Here's how the part is built. I have some questions about the finished solid (model axes, mm). Face numbers are marked on the shaded views. A direction names the side the tool comes from. Give positions to 0.01 mm unless a question says otherwise; leave off trailing zeros. Loops run counter-clockwise (first coordinate to the right, second up) from the corner with the lowest first, then second, coordinate; pieces in that order, holes last. Notation, with made-up numbers: (43, 35) - (65, 35) arc R14 cw to (65, 45) - close; hole circle Ø2 at (16.25, 76). An arc over 180 degrees is marked (long way). Use one line per item in the form item = value.
from build123d import *

# Parameters (mm, degrees)
SKETCH_2_R          = 23.5
EXTRUDE_1_DEPTH     = 50
FILLET_3_R          = 10
SHELL_2_T           = -2
SKETCH_5_R          = 9.5
EXTRUDE_2_DEPTH     = 48
SKETCH_6_R          = 2.4
CUT_EXTRUDE_1_DEPTH = 61.037488289
EXTRUDE_3_REACH     = 62.037
SKETCH_7_W          = 1.2
SKETCH_7_H          = 13
SKETCH_8_R          = 7.5
CUT_EXTRUDE_2_DEPTH = 39
CHAMFER_1_SIZE      = 3


with BuildPart() as part:
    # Эскиз2 → Бобышка-Вытянуть1 (new body)
    with BuildSketch(Plane.XY):
        Circle(SKETCH_2_R)
    extrude(amount=EXTRUDE_1_DEPTH)

    # Скругление3
    fillet_3_edges = [part.edges().sort_by_distance(p)[0] for p in [
        (-23.5, 0, 50),
    ]]
    fillet(fillet_3_edges, radius=FILLET_3_R)

    # Оболочка2
    shell_2_openings = [part.faces().sort_by_distance(p)[0] for p in [
        (0, 0, 0),
    ]]
    offset(amount=SHELL_2_T, openings=shell_2_openings, kind=Kind.INTERSECTION)

    # Эскиз5 → Бобышка-Вытянуть2 (add)
    with BuildSketch(Plane(origin=(0, 0, 48), x_dir=(-1, 0, 0), z_dir=(0, 0, -1))):
        with Locations(Location((0, 0, 0), (0, 0, 180))):
            Circle(SKETCH_5_R)
    extrude(amount=EXTRUDE_2_DEPTH)

    # Эскиз6 → Вырез-Вытянуть1 (cut, through all)
    with BuildSketch(Plane(origin=(0, 0, 0), x_dir=(-1, 0, 0), z_dir=(0, 0, -1))):
        Circle(SKETCH_6_R)
    extrude(amount=-CUT_EXTRUDE_1_DEPTH, mode=Mode.SUBTRACT)

    # Эскиз7 → Бобышка-Вытянуть3 (add, up to next)
    with BuildSketch(Plane(origin=(0, 0, 0), x_dir=(-1, 0, 0), z_dir=(0, 0, -1)), mode=Mode.PRIVATE) as extrude_3_sk1:
        with Locations((0, 15.437627965)):
            Rectangle(SKETCH_7_W, SKETCH_7_H)
    extrude_3_tool1 = extrude(extrude_3_sk1.sketch, amount=-EXTRUDE_3_REACH, mode=Mode.PRIVATE) - part.part
    # Эскиз7 → Бобышка-Вытянуть3 (add, up to next)
    with BuildSketch(Plane(origin=(0, 0, 0), x_dir=(-1, 0, 0), z_dir=(0, 0, -1)), mode=Mode.PRIVATE) as extrude_3_sk2:
        Polygon((7.440212867, 4.988429225), (18.698543116, 11.488429225), (19.298543116, 10.44919874), (8.040212867, 3.94919874), align=None)
    extrude_3_tool2 = extrude(extrude_3_sk2.sketch, amount=-EXTRUDE_3_REACH, mode=Mode.PRIVATE) - part.part
    # Эскиз7 → Бобышка-Вытянуть3 (add, up to next)
    with BuildSketch(Plane(origin=(0, 0, 0), x_dir=(-1, 0, 0), z_dir=(0, 0, -1)), mode=Mode.PRIVATE) as extrude_3_sk3:
        Polygon((8.040212867, -3.94919874), (19.298543117, -10.44919874), (18.698543117, -11.488429225), (7.440212867, -4.988429225), align=None)
    extrude_3_tool3 = extrude(extrude_3_sk3.sketch, amount=-EXTRUDE_3_REACH, mode=Mode.PRIVATE) - part.part
    # Эскиз7 → Бобышка-Вытянуть3 (add, up to next)
    with BuildSketch(Plane(origin=(0, 0, 0), x_dir=(-1, 0, 0), z_dir=(0, 0, -1)), mode=Mode.PRIVATE) as extrude_3_sk4:
        with Locations((0, -15.437627965)):
            Rectangle(SKETCH_7_W, SKETCH_7_H)
    extrude_3_tool4 = extrude(extrude_3_sk4.sketch, amount=-EXTRUDE_3_REACH, mode=Mode.PRIVATE) - part.part
    # Эскиз7 → Бобышка-Вытянуть3 (add, up to next)
    with BuildSketch(Plane(origin=(0, 0, 0), x_dir=(-1, 0, 0), z_dir=(0, 0, -1)), mode=Mode.PRIVATE) as extrude_3_sk5:
        Polygon((-7.440212867, -4.988429225), (-18.698543116, -11.488429225), (-19.298543116, -10.44919874), (-8.040212867, -3.94919874), align=None)
    extrude_3_tool5 = extrude(extrude_3_sk5.sketch, amount=-EXTRUDE_3_REACH, mode=Mode.PRIVATE) - part.part
    # Эскиз7 → Бобышка-Вытянуть3 (add, up to next)
    with BuildSketch(Plane(origin=(0, 0, 0), x_dir=(-1, 0, 0), z_dir=(0, 0, -1)), mode=Mode.PRIVATE) as extrude_3_sk6:
        Polygon((-8.040212867, 3.94919874), (-19.298543116, 10.44919874), (-18.698543116, 11.488429225), (-7.440212867, 4.988429225), align=None)
    extrude_3_tool6 = extrude(extrude_3_sk6.sketch, amount=-EXTRUDE_3_REACH, mode=Mode.PRIVATE) - part.part
    add(extrude_3_tool1.solids().sort_by_distance((0, 15.437628, 0))[0])
    add(extrude_3_tool2.solids().sort_by_distance((-13.369378, 7.718814, 0))[0])
    add(extrude_3_tool3.solids().sort_by_distance((-13.369378, -7.718814, 0))[0])
    add(extrude_3_tool4.solids().sort_by_distance((0, -15.437628, 0))[0])
    add(extrude_3_tool5.solids().sort_by_distance((13.369378, -7.718814, 0))[0])
    add(extrude_3_tool6.solids().sort_by_distance((13.369378, 7.718814, 0))[0])

    # Эскиз8 → Вырез-Вытянуть2 (cut)
    with BuildSketch(Plane.XY.offset(50)):
        Circle(SKETCH_8_R)
    extrude(amount=-CUT_EXTRUDE_2_DEPTH, mode=Mode.SUBTRACT)

    # Фаска1
    chamfer_1_edges = [part.edges().sort_by_distance(p)[0] for p in [
        (2.4, 0, 11),
    ]]
    chamfer(chamfer_1_edges, length=CHAMFER_1_SIZE)


solid = part.part
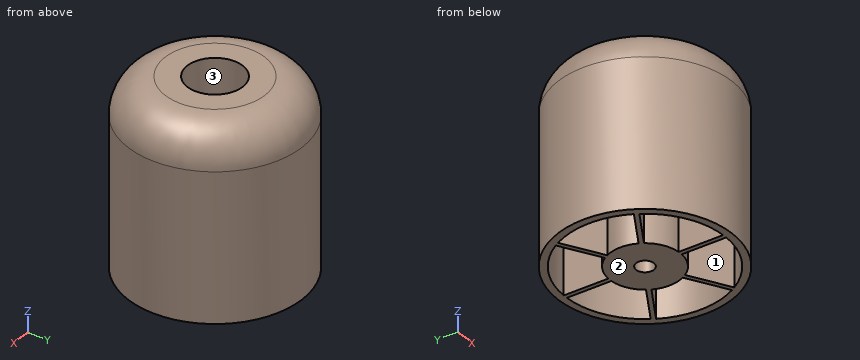
(1) If we section it at A-A (z = 21): List the corners of the cut face in (x, y) for me.
Geometry says:
outline = circle Ø47 at (0, 0); hole (-18.91, -10.23) - (-8.51, -4.22) arc R9.5 cw to (-8.51, 4.22) - (-18.91, 10.23) arc R21.5 ccw to start; hole (-18.31, -11.27) arc R21.5 ccw to (-0.6, -21.49) - (-0.6, -9.48) arc R9.5 cw to (-7.91, -5.26) - close; hole (-18.31, 11.27) - (-7.91, 5.26) arc R9.5 cw to (-0.6, 9.48) - (-0.6, 21.49) arc R21.5 ccw to start; hole circle Ø15 at (0, 0); hole (0.6, -21.49) arc R21.5 ccw to (18.31, -11.27) - (7.91, -5.26) arc R9.5 cw to (0.6, -9.48) - close; hole (0.6, 9.48) arc R9.5 cw to (7.91, 5.26) - (18.31, 11.27) arc R21.5 ccw to (0.6, 21.49) - close; hole (8.51, -4.22) - (18.91, -10.23) arc R21.5 ccw to (18.91, 10.23) - (8.51, 4.22) arc R9.5 cw to start
(2) If I drill on probe 1 along Y at (x, z) = (0, 5); probe 2 along Y at (x, z) = (0, 29.5); probe 3 along X at (y, z) = (-6, 16), over which ranges is the centre line in solid material (lowest first)?
Geometry says:
probe_1 = -23.5 to -2.4, 2.4 to 23.5
probe_2 = -23.5 to -7.5, 7.5 to 23.5
probe_3 = -22.72 to -20.65, -11.59 to -9.19, -7.37 to -4.5, 4.5 to 7.37, 9.19 to 11.59, 20.65 to 22.72
(3) If we section it at B-B (y = 0): List the corners of the cut face in (x, z) for me, plus the area to 3 significant figures.
Geometry says:
outline = (-23.5, 0) - (-21.5, 0) - (-21.5, 40) arc R8 cw to (-13.5, 48) - (-9.5, 48) - (-9.5, 0) - (-2.4, 0) - (-2.4, 8) - (-5.4, 11) - (-7.5, 11) - (-7.5, 50) - (-13.5, 50) arc R10 ccw to (-23.5, 40) - close; (2.4, 0) - (9.5, 0) - (9.5, 48) - (13.5, 48) arc R8 cw to (21.5, 40) - (21.5, 0) - (23.5, 0) - (23.5, 40) arc R10 ccw to (13.5, 50) - (7.5, 50) - (7.5, 11) - (5.4, 11) - (2.4, 8) - close
area = 536 mm²
(4) For the marked faces 1, 2 and 3, which set-ups out of +Z, -Z, +X, -X, +Y, -Y let a thin tool reach every point of the face, with its end or its side?
Geometry says:
face_1 = -Z
face_2 = -Z, +X, -X, +Y, -Y
face_3 = +Z
(5) For P1, Ø12, axis at x = 18.5, z = 17.5, coming from the -Y side; P2, Ø9.5, axis at y = 17, z = 13.5, coming from the -X side; P3, Ø5, axis at x = 6.5, z = 40.5, coming from the +Y side; P4, Ø4.5, axis at x = 0, y = 0, coming from the -Z side, each with a flat end and sliding along its axis, tell me the tip position at first contact or that it passes through.
Geometry says:
P1 = -19.9
P2 = -20.05
P3 = 23.15
P4 = through
